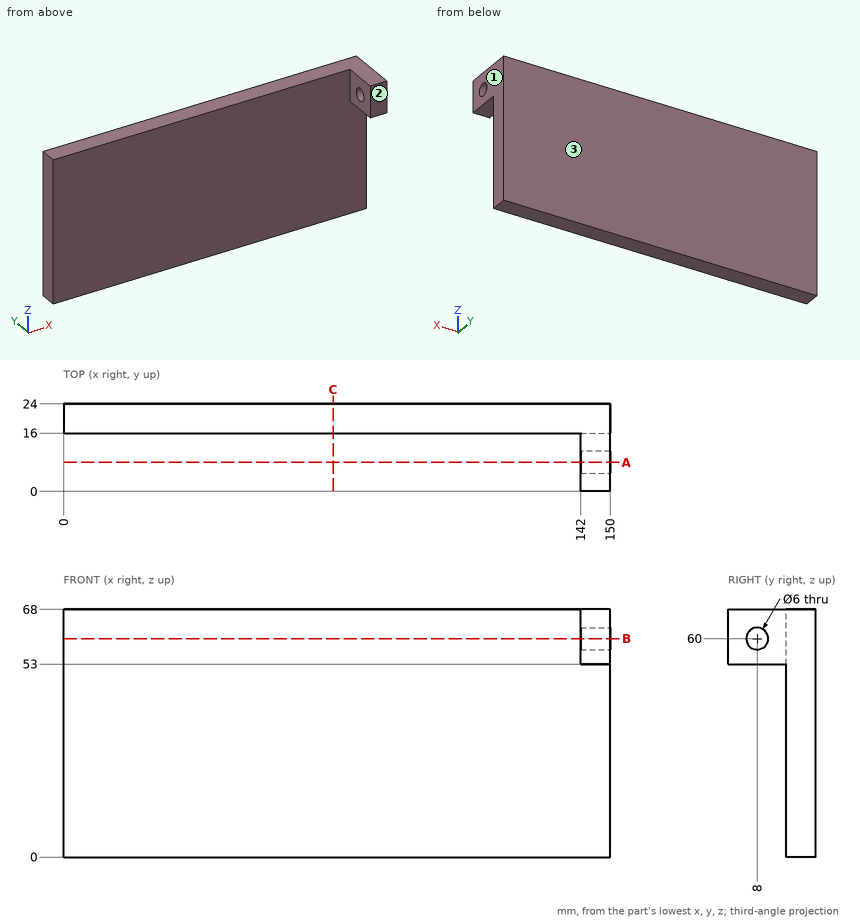
Check sheet for the drawn part. Datum: minimum x, y, z corner. Units: mm. Round coordinates to 2 decimals unless told otherwise and drop trailing zeros. Loops run counter-clockwise (first coordinate to the right, second up) from the corner with the lowest first, then second, coordinate; pieces in that order, holes last. Notation, with made-up numbers: (25, -13.5) - (29, -13.5) arc R6 cw to (29, -6.5) - close; hole circle Ø5 at (-0.5, -7.75). An arc over 180 degrees is marked (long way). Write item = value, one per line. Start each with the question number.
1. Section check B-B on z = 60. Enter the section's corners in (x, y).
2. Mould release check, pull along Y, two halves, no side actions. Record for the marked faces 1, 2 and 3: released by +Y, released by -Y, zero draft, split by the parting line, or undercut.
3. Depth check by flat-ended pin: pin 1 (12 mm diameter, centred on y = 8.5, z = 20, fed in from +X) (3 decimals); pin 2 (12 mm diameter, centred on y = 8, z = 58, fed in from -X); pin 3 (20.5 mm diameter, centred on x = 41.5, z = 42, fed in from -Y); pin 4 (6.5 mm diameter, centred on x = 145, y = 6.5, fed in from -Z). Enter the tip coordinate at first touch or a pass-through.
4. Section check C-C on x = 74. Enter the section's corners in (y, z).
5. Thickness scan on line 1 (Z direction, x = 145.5, y = 8); line 2 (Y direction, x = 106, z = 52.5); line 3 (X direction, y = 3.5, z = 58.5). Record the ranges inside material, lowest first.
6. Section check A-A on y = 8. Enter the section's corners in (x, z), then the cut area to 3 significant figures.
Working result:
q1.outline = (0, 16) - (142, 16) - (142, 11) - (150, 11) - (150, 24) - (0, 24) - close; (142, 0) - (150, 0) - (150, 5) - (142, 5) - close
q2.face_1 = zero draft
q2.face_2 = released by -Y
q2.face_3 = released by +Y
q3.pin_1 = through
q3.pin_2 = 142
q3.pin_3 = 16
q3.pin_4 = 53
q4.outline = (16, 0) - (24, 0) - (24, 68) - (16, 68) - close
q5.line_1 = 53 to 57, 63 to 68
q5.line_2 = 16 to 24
q5.line_3 = 142 to 150
q6.outline = (142, 53) - (150, 53) - (150, 57) - (142, 57) - close; (142, 63) - (150, 63) - (150, 68) - (142, 68) - close
q6.area = 72.0 mm^2
